Work out the finished part from the listing and answer in its coordinate system (mm). Face numbers are marked on the shaded views. A direction names the side the tool comes from. Round coordinates to 2 decimals unless told otherwise and drop trailing zeros. Order: outer loops, then holes, each group sorted by start corner. A loop starts at its lowest first (then second) coordinate and runs counter-clockwise, first axis right, second up. Notation, with made-up numbers: (27, -36.5) - (51, -36.5) arc R17 cw to (51, -20.5) - close; hole circle Ø1 at (-1, 17). An arc over 180 degrees is marked (long way). Use CSV: the item, a comma, the result in double quotes.
from build123d import *

# Parameters (mm, degrees)
SKETCH2_R           = 2.75
BOSS_EXTRUDE2_DEPTH = 35
CUT_EXTRUDE1_DEPTH  = 35
CUT_EXTRUDE2_DEPTH  = 35


with BuildPart() as part:
    # Sketch2 → Boss-Extrude2 (new body)
    with BuildSketch(Plane(origin=(0, 0, 0), x_dir=(1, 0, 0), z_dir=(0, 1, 0))):
        with BuildLine():
            Line((7.5, 3.904252879), (7.5, 75))
            ThreePointArc((7.5, 75), (0, 82.5), (-7.5, 75))
            Line((-7.5, 75), (-7.5, 0))
            ThreePointArc((-7.5, 0), (-6.652581249, -3.463114599), (-4.301823273, -6.143640332))
            Line((-4.301823273, -6.143640332), (20.272738056, -23.350933423))
            ThreePointArc((20.272738056, -23.350933423), (30.718201661, -21.509116363), (28.876384601, -11.063652758))
            Line((28.876384601, -11.063652758), (7.5, 3.904252879))
        make_face()
        Circle(SKETCH2_R, mode=Mode.SUBTRACT)
        with Locations((0, 75)):
            Circle(SKETCH2_R, mode=Mode.SUBTRACT)
        with Locations((24.574561329, -17.207293091)):
            Circle(SKETCH2_R, mode=Mode.SUBTRACT)
    extrude(amount=BOSS_EXTRUDE2_DEPTH)

    # Sketch3 → Cut-Extrude1 (cut)
    with BuildSketch(Plane(origin=(7.5, 0, 0), x_dir=(0, 0, -1), z_dir=(1, 0, 0))):
        Polygon((75, 12), (65, 12), (65, 23), (87.183204073, 23), (87.183204073, 12), align=None)
    extrude(amount=-CUT_EXTRUDE1_DEPTH, mode=Mode.SUBTRACT)

    # Sketch4 → Cut-Extrude2 (cut)
    with BuildSketch(Plane(origin=(4.301823273, 0, -6.143640332), x_dir=(-0.819152044, 0, -0.573576436), z_dir=(0.573576436, 0, -0.819152044))):
        Polygon((-30, 12), (-30, 17.5), (-30, 23), (-43.630298532, 23), (-43.630298532, 12), align=None)
        Polygon((-30, 23), (-30, 17.5), (-30, 12), (-20, 12), (-20, 23), align=None)
    extrude(amount=-CUT_EXTRUDE2_DEPTH, mode=Mode.SUBTRACT)


solid = part.part
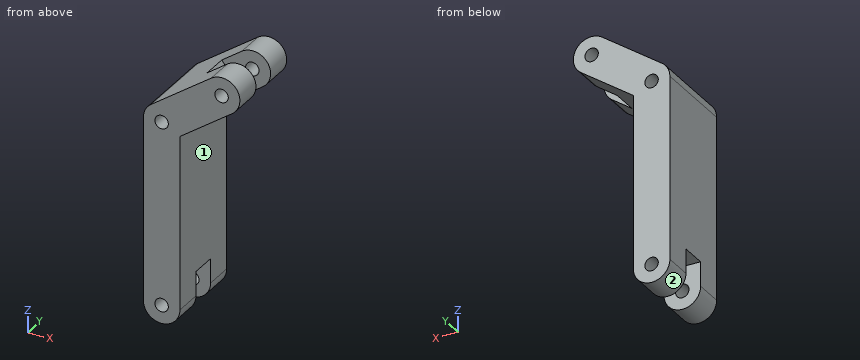
(1) For the marked faces 1 and 2, determine the directions among +Z, -Z, +X, -X, +Y, -Y from which every point of the face is accessible in a straight line to the end or side of a thin tool.
Findings below:
face 1,"-Z, +X, +Y, -Y"
face 2,"-Z, +Y, -Y"
(2) Find the intervals of material crossed by L1, parallel to X at y = 7.25, z = -75; L2, parallel to Z at x = -0.5, y = 9; L3, parallel to Z at x = 0, y = 9, in increasing order. Write a range as from..to.
Findings below:
L1,"x = -7.5..-2.75, 2.75..7.5"
L2,"z = -82.48..-77.7, -72.3..-2.7, 2.7..8.81"
L3,"z = -82.5..-77.75, -72.25..-2.75, 2.75..9.16"
(3) Find section B-B (x = 0). Determine the outline of the cut face in (y, z).
Findings below:
outline,"(0, -82.5) - (12, -82.5) - (12, -77.75) - (0, -77.75) - close; (0, -72.25) - (12, -72.25) - (12, -65) - (23, -65) - (23, -72.25) - (35, -72.25) - (35, -2.75) - (0, -2.75) - close; (0, 2.75) - (35, 2.75) - (35, 9.16) - (0, 9.16) - close; (23, -82.5) - (35, -82.5) - (35, -77.75) - (23, -77.75) - close"
(4) Find section C-C (y = 9.5). Determine the outline of the cut face in (x, z).
Findings below:
outline,"(-7.5, -75) arc R7.5 ccw to (7.5, -75) - (7.5, -3.9) - (28.88, 11.06) arc R7.5 ccw to (20.27, 23.35) - (-4.3, 6.14) arc R7.5 ccw to (-7.5, 0) - close; hole circle Ø5.5 at (0, -75); hole circle Ø5.5 at (0, 0); hole circle Ø5.5 at (24.57, 17.21)"
(5) Each of these flat-tipped pins is pushed along its axis until it touches: pin 1 (17.5 mm diameter, centred on y = 10, z = -47.5, fed in from +X); pin 2 (4 mm diameter, centred on x = 20, y = 5.5, fed in from +Z); pin 3 (4 mm diameter, centred on y = 23, z = 6, fed in from +X); pin 4 (5 mm diameter, centred on x = 24.57, z = 17.21, fed in from -Y). Where does it stop, or does it pass through?
Findings below:
pin 1,"stops at x = 7.5"
pin 2,"stops at z = 24.25"
pin 3,"stops at x = 24.5"
pin 4,"passes through"
(6) Find section D-D (z = -49.5). Determine the outline of the cut face in (x, y), and give its area (3 significant figures).
Findings below:
outline,"(-7.5, 0) - (7.5, 0) - (7.5, 35) - (-7.5, 35) - close"
area,"525 mm²"
(7) Find section A-A (y = 16). Determine the outline of the cut face in (x, z), and give its area (3 significant figures).
Findings below:
outline,"(-7.5, -65) - (7.5, -65) - (7.5, -3.9) - (20.68, 5.33) - (12.08, 17.62) - (-4.3, 6.14) arc R7.5 ccw to (-7.5, 0) - close; hole circle Ø5.5 at (0, 0)"
area,"1,250 mm²"
